Geometry check sheet. Reference: the model listing, model coordinates, mm. A direction names the side the tool comes from. Coordinates: 2 decimals unless noted, no trailing zeros. Write each loop counter-clockwise with the first axis right and the second up, starting at its lowest first coordinate (ties: lowest second). Pieces come first, ordered by that corner, then holes. Notation, with made-up numbers: M 20,18 L 54,18 A19 ccw 54,30 Z; hole C 43.25,-26.75 d3. An arc over 180 degrees is marked long. Put each result on its own line as item: value. Start each with the question number.
1) Scan lines: line 1 along Y through (x, z) = (-32, -2.25); line 2 along Y through (x, z) = (48.5, 0.5); line 3 along X through (y, z) = (31, -4). Record each from-to range of solid material in increasing order.
2) Cross-section at A-A on z = -0.25. Record the cut outline in (x, y).
3) Cross-section at C-C on y = -11.5. Record the cut outline in (x, z).
4) Cross-section at B-B on y = 31.75. Record the cut outline in (x, z) (3 decimals).
5) Gauge pin test, flat ends, axial feed: pin 1 (6 mm diameter, centred on x = -101.5, z = 3.5, fed in from +Y); pin 2 (6 mm diameter, centred on x = 92, z = -3, fed in from +Y); pin 3 (1.5 mm diameter, centred on x = -92, z = -1.5, fed in from -Y). Record the tip position at first contact, or that the pin passes through.
6) Set-up check for faces 5 (the cylindrical face through (-50.8, 31.6, 0.1)), 6 (the flat face through (101.067, 25.756, 0.071)): record each of +Z, -Z, +X, -X, +Y, -Y from which the full face is reachable in a straight line by a thin tool's end or side.
7) Mould release check, pull along Y, two halves, no side actions. Record for faces 1 (the flat face through (1, -50.8, 0)), 2 (the flat face through (2, 1, 5.08)), 3 (the cylindrical face through (50.8, 31.9, 0.1)), 4 (the flat face through (-1, 38.1, 0)): released by +Y, released by -Y, zero draft, split by the parting line, or undercut.
8) Cross-section at D-D on x = 117. Record the cut outline in (y, z), plus the area to 3 significant figures.
from build123d import *

# Parameters (mm, degrees)
BOSS_EXTRUDE1_DEPTH = 5.08


with BuildPart() as part:
    # Sketch1 → Boss-Extrude1 (new, symmetric)
    with BuildSketch(Plane.XY):
        Polygon((-63.5, 50.8), (63.5, 50.8), (139.7, 0), (63.5, -50.8), (-63.5, -50.8), (-139.7, 0), align=None)
        with BuildLine():
            Line((-44.45, 38.1), (44.45, 38.1))
            ThreePointArc((44.45, 38.1), (50.8, 31.75), (44.45, 25.4))
            Line((44.45, 25.4), (-44.45, 25.4))
            ThreePointArc((-44.45, 25.4), (-50.8, 31.75), (-44.45, 38.1))
        make_face(mode=Mode.SUBTRACT)
    extrude(amount=BOSS_EXTRUDE1_DEPTH, both=True)


solid = part.part
Answer key:
1. line 1: y = -50.8 to 25.4, 38.1 to 50.8
1. line 2: y = -50.8 to 26.86, 36.64 to 50.8
1. line 3: x = -93.2 to -50.76, 50.76 to 93.2
2. outline: M -139.7,0 L -63.5,-50.8 L 63.5,-50.8 L 139.7,0 L 63.5,50.8 L -63.5,50.8 Z; hole M -44.45,25.4 L 44.45,25.4 A6.35 ccw 44.45,38.1 L -44.45,38.1 A6.35 ccw Z
3. outline: M -122.45,-5.08 L 122.45,-5.08 L 122.45,5.08 L -122.45,5.08 Z
4. outline: M -92.075,-5.08 L -50.8,-5.08 L -50.8,5.08 L -92.075,5.08 Z; M 50.8,-5.08 L 92.075,-5.08 L 92.075,5.08 L 50.8,5.08 Z
5. pin 1: stops at y = 27.47
5. pin 2: stops at y = 33.8
5. pin 3: stops at y = -32.3
6. face 5: +Z, -Z
6. face 6: +Z, -Z, +X, +Y
7. face 1: released by -Y
7. face 2: zero draft
7. face 3: undercut
7. face 4: undercut
8. outline: M -15.13,-5.08 L 15.13,-5.08 L 15.13,5.08 L -15.13,5.08 Z
8. area: 308 mm²
